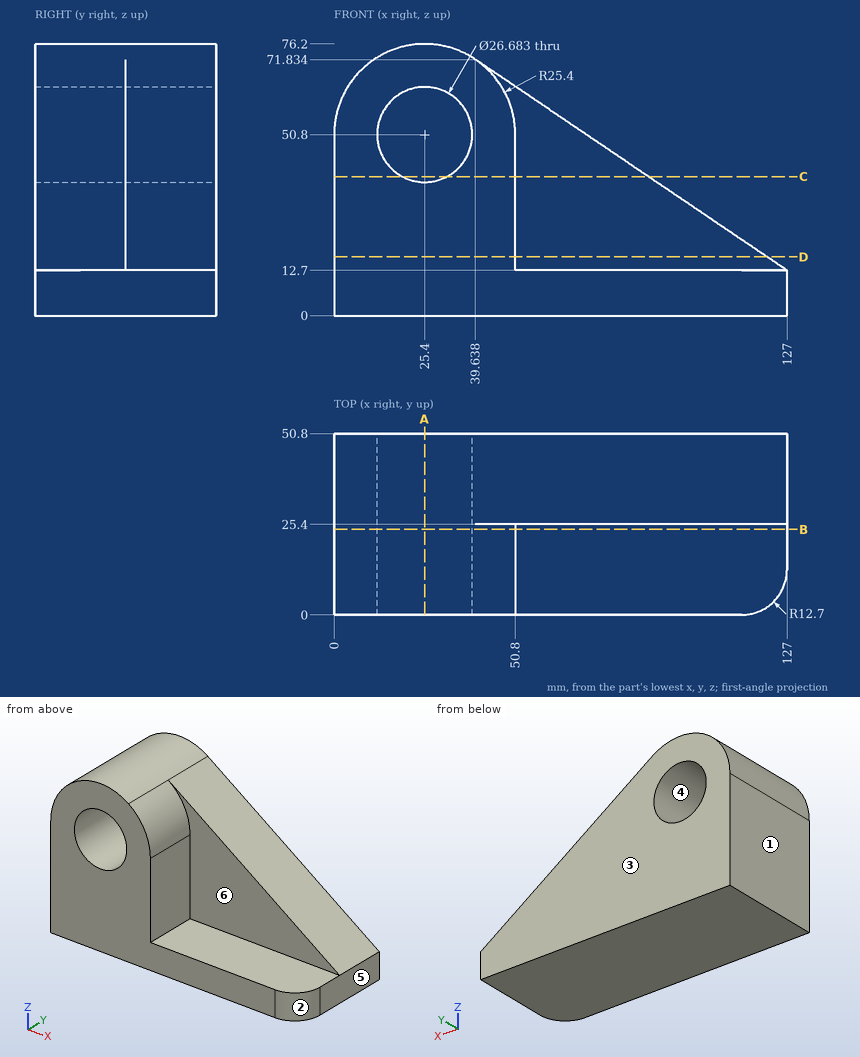
The drawing under review shows one solid part. Ordinate dimensions are in mm from its lowest x, y, z. A direction names the side the tool comes from. Round coordinates to 2 decimals unless told otherwise and drop trailing zeros. Write each loop counter-clockwise with the first axis right and the second up, starting at its lowest first coordinate (ties: lowest second). Pieces come first, ordered by that corner, then holes.
(1) Wall thickness on L1, parallel to Z at x = 25.4, y = 38; L2, parallel to X at y = 22, z = 50; L3, parallel to X at y = 3.5, z = 29.5: over which ranges is each line inside the solid? List them lowest first.
(2) We need section A-A on x = 25.4. Give the boundary of the cut face in (y, z), and give its area (3 significant figures).
(3) Mouldability with a two-part tool opening along X and no side actions: class the marked faces 1, 2, 3 and 4 as +X half, -X half, draft (parallel to the pull), parting line (faces both ways), or undercut.
(4) We need section D-D on z = 16.5. Give the boundary of the cut face in (x, y).
(5) We need section B-B on y = 24. Give the boundary of the cut face in (x, z) (1 decimal).
(6) We need section C-C on z = 39. Give the boundary of the cut face in (x, y) (1 decimal).
(7) Machinability: for the marked faces 5 and 6, which of the approach directions +Z, -Z, +X, -X, +Y, -Y give a long, thin tool a straight path to every point of the face, cutting with its end or side? Answer none if there is none.
(8) Insertion check: pin 1 (2 mm diameter, centred on x = 44, y = 28, fed in from +Z); pin 2 (4 mm diameter, centred on x = 58.5, y = 10.5, fed in from -Z); pin 3 (1 mm diameter, centred on x = 112, z = 23, fed in from -Y); pin 4 (5 mm diameter, centred on y = 19.5, z = 45.5, fed in from +X). Each pin has a flat end and moves straight along its axis. Give the tip position at first contact, or say it passes through.
Findings below:
1. L1: z = 0 to 37.46, 64.14 to 76.2
1. L2: x = 0 to 12.08, 38.72 to 50.8
1. L3: x = 0 to 50.8
2. outline: (0, 0) - (50.8, 0) - (50.8, 37.46) - (0, 37.46) - close; (0, 64.14) - (50.8, 64.14) - (50.8, 76.2) - (0, 76.2) - close
2. area: 2,520 mm2
3. face 1: -X half
3. face 2: +X half
3. face 3: draft
3. face 4: undercut
4. outline: (0, 0) - (50.8, 0) - (50.8, 25.4) - (121.39, 25.4) - (121.39, 50.8) - (0, 50.8) - close
5. outline: (0, 0) - (127, 0) - (127, 12.7) - (50.8, 12.7) - (50.8, 50.8) arc R25.4 ccw to (39.6, 71.8) arc R25.4 ccw to (0, 50.8) - close; hole circle Ø26.7 at (25.4, 50.8)
6. outline: (0, 0) - (19.2, 0) - (19.2, 50.8) - (0, 50.8) - close; (31.6, 0) - (50.8, 0) - (50.8, 25.4) - (88.1, 25.4) - (88.1, 50.8) - (31.6, 50.8) - close
7. face 5: +Z, -Z, +X, +Y, -Y
7. face 6: +Z, +X, -Y
8. pin 1: stops at z = 69.56
8. pin 2: stops at z = 0
8. pin 3: stops at y = 25.4
8. pin 4: stops at x = 50.8
